Model file for the job. Use its own axes, mm. Face numbers are marked on the shaded views. Give positions to 0.01 mm unless a question says otherwise; leave off trailing zeros. Write each loop counter-clockwise with the first axis right and the second up, starting at its lowest first coordinate (ties: lowest second). Pieces come first, ordered by that corner, then holes. Notation, with made-up numbers: M 36,23.5 L 71,23.5 A27 cw 71,44.5 Z; hole C -21,46 d2. An arc over 180 degrees is marked long. Answer as a JSON object with one key per item and string values. Group by question number.
```python
from build123d import *

# Parameters (mm, degrees)
SKETCH1_W           = 63.5
SKETCH1_H           = 168
BOSS_EXTRUDE1_DEPTH = 9.525
SKETCH4_W           = 63.5
SKETCH4_H           = 12
BOSS_EXTRUDE2_DEPTH = 6
SKETCH6_R           = 2
CUT_EXTRUDE1_DEPTH  = 181.270007558
SKETCH8_R           = 0.877320143
CUT_EXTRUDE4_DEPTH  = 180.852649758


with BuildPart() as part:
    # Sketch1 → Boss-Extrude1 (new body)
    with BuildSketch(Plane.XY):
        with Locations((31.75, 84)):
            Rectangle(SKETCH1_W, SKETCH1_H)
    extrude(amount=BOSS_EXTRUDE1_DEPTH)

    # Sketch4 → Boss-Extrude2 (add)
    with BuildSketch(Plane(origin=(0, 0, 0), x_dir=(-1, 0, 0), z_dir=(0, 0, -1))):
        with Locations((-31.75, 162)):
            Rectangle(SKETCH4_W, SKETCH4_H)
    boss_extrude2 = extrude(amount=BOSS_EXTRUDE2_DEPTH)

    # Sketch6 → Cut-Extrude1 (cut, through all)
    with BuildSketch(Plane(origin=(0, 0, -6), x_dir=(-1, 0, 0), z_dir=(0, 0, -1))):
        with Locations((-5.74011002, 164)):
            Circle(SKETCH6_R)
        with Locations((-53.74011002, 164)):
            Circle(SKETCH6_R)
        with Locations((-29.74011002, 164)):
            Circle(SKETCH6_R)
    cut_extrude1 = extrude(amount=-CUT_EXTRUDE1_DEPTH, mode=Mode.SUBTRACT)

    # Mirror1: Boss-Extrude2, Cut-Extrude1 across plane
    add(boss_extrude2.mirror(Plane.ZX.offset(84)))
    add(cut_extrude1.mirror(Plane.ZX.offset(84)), mode=Mode.SUBTRACT)

    # Sketch8 → Cut-Extrude4 (cut, symmetric)
    with BuildSketch(Plane(origin=(0, 0, 0), x_dir=(-1, 0, 0), z_dir=(0, 0, -1))):
        with Locations((-14.479670844, 130.185691353)):
            Circle(SKETCH8_R)
        with Locations((-25.479670844, 130.185691353)):
            Circle(SKETCH8_R)
        with Locations((-36.479670844, 130.185691353)):
            Circle(SKETCH8_R)
    cut_extrude4 = extrude(amount=CUT_EXTRUDE4_DEPTH, both=True, mode=Mode.SUBTRACT)

    # Mirror2: Cut-Extrude4 across plane
    add(cut_extrude4.mirror(Plane.ZX.offset(84)), mode=Mode.SUBTRACT)


solid = part.part
```
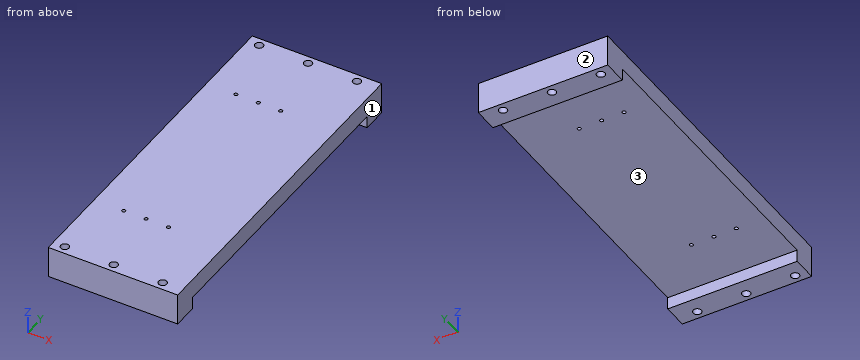
Q1. Wall check: L1, parallel to X at y = 4, z = 3.75; L2, parallel to Y at x = 25.5, z = 4.75; L3, parallel to Y at x = 27, z = -3.5. Give the ranges that are in metal, low to high.
Q2. Slice it at B-B, the plane y = 164. Write the cut outline in (x, z) (3 decimals).
Q3. Slice it at A-A, the plane z = -2.5. Write the cut outline in (x, y).
Q4. Slice it at D-D, the plane y = 64.5. Write the cut outline in (x, z) (3 decimals).
Q5. Drop a flat-ended pin along its axis: P1, Ø2.5, axis at x = 25.48, y = 37.81, coming from the -Z side. Give the stop position or say it passes through.
Q6. Two-plate mould, pull along Y, no slides. Class the marked faces 1, 2 and 3: +Y half, -Y half, draft (parallel to the pull), parting line (faces both ways), or undercut.
Q7. Slice it at C-C, the plane x = 49. Write the cut outline in (y, z) (3 decimals), then the cut area to 3 significant figures.
Solved:
{
 "1": {"L1": "x = 0 to 3.74, 7.74 to 27.74, 31.74 to 51.74, 55.74 to 63.5", "L2": "y = 0 to 36.94, 38.69 to 129.31, 131.06 to 168", "L3": "y = 0 to 12, 156 to 168"},
 "2": {"outline": "M 0,-6 L 3.74,-6 L 3.74,9.525 L 0,9.525 Z; M 7.74,-6 L 27.74,-6 L 27.74,9.525 L 7.74,9.525 Z; M 31.74,-6 L 51.74,-6 L 51.74,9.525 L 31.74,9.525 Z; M 55.74,-6 L 63.5,-6 L 63.5,9.525 L 55.74,9.525 Z"},
 "3": {"outline": "M 0,0 L 63.5,0 L 63.5,12 L 0,12 Z; M 0,156 L 63.5,156 L 63.5,168 L 0,168 Z; hole C 5.74,4 d4; hole C 5.74,164 d4; hole C 29.74,4 d4; hole C 29.74,164 d4; hole C 53.74,4 d4; hole C 53.74,164 d4"},
 "4": {"outline": "M 0,0 L 63.5,0 L 63.5,9.525 L 0,9.525 Z"},
 "5": {"P1": "stops at z = 0"},
 "6": {"face 1": "draft", "face 2": "+Y half", "face 3": "undercut"},
 "7": {"outline": "M 0,-6 L 12,-6 L 12,0 L 156,0 L 156,-6 L 168,-6 L 168,9.525 L 0,9.525 Z", "area": "1,740 mm²"}
}
